from build123d import *

# Parameters (mm, degrees)
SKETCH10_R              = 7.4
SKETCH10_R_2            = 4.5
BOSS_EXTRUDE3_DEPTH     = 1.2
SKETCH11_R              = 7.4
SKETCH11_R_2            = 5.2
BOSS_EXTRUDE4_DEPTH     = 20
BOSS_EXTRUDE5_DEPTH     = 7
SKETCH12_R              = 0.75
CUT_EXTRUDE1_DEPTH      = 10
CUT_EXTRUDE1_DEPTH_BACK = 11
SKETCH14_W              = 4.2
SKETCH14_H              = 1
CUT_EXTRUDE2_DEPTH      = 6
CUT_EXTRUDE3_REACH      = 29.148
CUT_EXTRUDE3_END_RADIUS = 7.4
CUT_EXTRUDE6_DEPTH      = 1
SKETCH16_R              = 0.8
CUT_EXTRUDE4_DEPTH      = 10
CUT_EXTRUDE4_DEPTH_BACK = 10
SKETCH19_R              = 7.4
SKETCH19_R_2            = 7
CUT_EXTRUDE7_DEPTH      = 15.2
FILLET1_R               = 1


with BuildPart() as part:
    # Sketch10 → Boss-Extrude3 (new body)
    with BuildSketch(Plane.XY):
        Circle(SKETCH10_R)
        Circle(SKETCH10_R_2, mode=Mode.SUBTRACT)
    extrude(amount=BOSS_EXTRUDE3_DEPTH)

    # Sketch11 → Boss-Extrude4 (add)
    with BuildSketch(Plane(origin=(0, 0, 0), x_dir=(-1, 0, 0), z_dir=(0, 0, -1))):
        Circle(SKETCH11_R)
        Circle(SKETCH11_R_2, mode=Mode.SUBTRACT)
    extrude(amount=BOSS_EXTRUDE4_DEPTH)

    # Sketch13 → Boss-Extrude5 (add)
    with BuildSketch(Plane.XY.offset(1.2)):
        with BuildLine():
            ThreePointArc((-2.9, 6.808083431), (0, 7.4), (2.9, 6.808083431))
            Line((2.9, 6.808083431), (2.9, 8.4))
            Line((2.9, 8.4), (-2.9, 8.4))
            Line((-2.9, 8.4), (-2.9, 6.808083431))
        make_face()
        with BuildLine():
            ThreePointArc((2.9, -6.808083431), (0, -7.4), (-2.9, -6.808083431))
            Line((-2.9, -6.808083431), (-2.9, -8.4))
            Line((-2.9, -8.4), (2.9, -8.4))
            Line((2.9, -8.4), (2.9, -6.808083431))
        make_face()
    extrude(amount=-BOSS_EXTRUDE5_DEPTH)

    # Sketch12 → Cut-Extrude1 (cut, two sides)
    with BuildSketch(Plane(origin=(0, 0, 0), x_dir=(1, 0, 0), z_dir=(0, 1, 0))) as cut_extrude1_sk:
        with Locations(Location((0, 1.8, 0), (0, 0, 90))):
            Circle(SKETCH12_R)
    extrude(amount=CUT_EXTRUDE1_DEPTH, mode=Mode.SUBTRACT)
    extrude(cut_extrude1_sk.sketch, amount=-CUT_EXTRUDE1_DEPTH_BACK, mode=Mode.SUBTRACT)

    # Sketch14 → Cut-Extrude2 (cut)
    with BuildSketch(Plane.XY.offset(1.2)):
        with Locations((0, 7.9)):
            Rectangle(SKETCH14_W, SKETCH14_H)
        with Locations((0, -7.9)):
            Rectangle(SKETCH14_W, SKETCH14_H)
    extrude(amount=-CUT_EXTRUDE2_DEPTH, mode=Mode.SUBTRACT)

    # Cut-Extrude3: up to this cylinder (the profile starts outside it)
    cut_extrude3_end = Plane(origin=(0, 0, -5.3), z_dir=(0, 0, -1)) * Cylinder(CUT_EXTRUDE3_END_RADIUS, 74.096, mode=Mode.PRIVATE)
    # Sketch15 → Cut-Extrude3 (cut, up to the surface)
    with BuildSketch(Plane(origin=(0, 8.4, 0), x_dir=(1, 0, 0), z_dir=(0, 1, 0)), mode=Mode.PRIVATE) as cut_extrude3_sk1:
        Polygon((-2.9, 5.8), (-2.9, 4.8), (-2.1, 4.8), (2.1, 4.8), (2.9, 4.8), (2.9, 5.8), align=None)
    cut_extrude3_tool1 = extrude(cut_extrude3_sk1.sketch, amount=-CUT_EXTRUDE3_REACH, mode=Mode.PRIVATE) - cut_extrude3_end
    add(cut_extrude3_tool1.solids().sort_by_distance((0, 8.4, -5.3))[0], mode=Mode.SUBTRACT)

    # Sketch18 → Cut-Extrude6 (cut)
    with BuildSketch(Plane(origin=(0, 0, -5.8), x_dir=(-1, 0, 0), z_dir=(0, 0, -1))):
        with BuildLine():
            Line((-2.9, -6.808083431), (-2.9, -8.4))
            Line((-2.9, -8.4), (2.9, -8.4))
            Line((2.9, -8.4), (2.9, -6.808083431))
            ThreePointArc((2.9, -6.808083431), (0, -7.4), (-2.9, -6.808083431))
        make_face()
    extrude(amount=-CUT_EXTRUDE6_DEPTH, mode=Mode.SUBTRACT)

    # Sketch16 → Cut-Extrude4 (cut, two sides)
    with BuildSketch(Plane(origin=(0, 0, 0), x_dir=(0, 0, -1), z_dir=(1, 0, 0))) as cut_extrude4_sk:
        with Locations(Location((15, 0, 0), (0, 0, 180))):
            Circle(SKETCH16_R)
    extrude(amount=CUT_EXTRUDE4_DEPTH, mode=Mode.SUBTRACT)
    extrude(cut_extrude4_sk.sketch, amount=-CUT_EXTRUDE4_DEPTH_BACK, mode=Mode.SUBTRACT)

    # Sketch19 → Cut-Extrude7 (cut)
    with BuildSketch(Plane(origin=(0, 0, -20), x_dir=(-1, 0, 0), z_dir=(0, 0, -1))):
        Circle(SKETCH19_R)
        Circle(SKETCH19_R_2, mode=Mode.SUBTRACT)
    extrude(amount=-CUT_EXTRUDE7_DEPTH, mode=Mode.SUBTRACT)

    # Fillet1
    fillet1_edges = [part.edges().sort_by_distance(p)[0] for p in [
        (7, 0, -20),
    ]]
    fillet(fillet1_edges, radius=FILLET1_R)


solid = part.part
Check sheet for the modelled part. Datum: model origin and axes. Units: mm. A direction names the side the tool comes from. Round coordinates to 2 decimals unless told otherwise and drop trailing zeros. Loops run counter-clockwise (first coordinate to the right, second up) from the corner with the lowest first, then second, coordinate; pieces in that order, holes last.
1. Sectioned sample at C-C on y = 0. Record the boundary of the cut face in (x, z), and give its area (3 significant figures).
2. Mould release check, pull along X, two halves, no side actions. Record for faces 6 (the cylindrical face through (-0.59, 4.46, 0.59)), 7 (the flat face through (-2.9, 8, -2)), 8 (the flat face through (2.9, 8, -2)), 9 (the flat face through (2, 5, -20)): released by +X, released by -X, zero draft, split by the parting line, or undercut.
3. Sectioned sample at B-B on z = -1.8. Record the boundary of the cut face in (x, y).
4. Set-up check for faces 1 (the flat face through (-2.1, -8, -2)), 2 (the flat face through (2.9, -8, -2)), 3 (the flat face through (-2.1, 8, -2)), 4 (the flat face through (-2.9, -8, -2)), 5 (the cylindrical face through (-4.96, 1.56, -9.86)): record each of +Z, -Z, +X, -X, +Y, -Y from which the full face is reachable in a straight line by a thin tool's end or side.
5. Gauge pin test, flat ends, axial feed: pin 1 Ø3.5 at (x, z) = (1, -1.5) entering from -Y; pin 2 Ø1.3 at (y, z) = (7.5, -3) entering from -X; pin 3 Ø0.8 at (y, z) = (7.5, -0.5) entering from +X; pin 4 Ø1.7 at (x, z) = (0, -1.8) entering from +Y. Record the tip position at first contact, or that the pin passes through.
6. Sectioned sample at A-A on x = 0. Record the boundary of the cut face in (y, z), and give its area (3 significant figures).
7. Sectioned sample at D-D on z = -4.5. Record the boundary of the cut face in (x, y).
8. Scan lines: probe 1 along Y at (x, z) = (0, 0.35); probe 2 along Y at (x, z) = (0, -4.5); probe 3 along Z at (x, y) = (4, 3). Record each from-to range of solid material in increasing order.
Recorded:
1. outline: (-7.4, -4.8) - (-7, -4.8) - (-7, -14.2) - (-5.2, -14.2) - (-5.2, 0) - (-4.5, 0) - (-4.5, 1.2) - (-7.4, 1.2) - close; (-7, -19) arc R1 ccw to (-6, -20) - (-5.2, -20) - (-5.2, -15.8) - (-7, -15.8) - close; (4.5, 0) - (5.2, 0) - (5.2, -14.2) - (7, -14.2) - (7, -4.8) - (7.4, -4.8) - (7.4, 1.2) - (4.5, 1.2) - close; (5.2, -20) - (6, -20) arc R1 ccw to (7, -19) - (7, -15.8) - (5.2, -15.8) - close
1. area: 76.6 mm2
2. face 6: undercut
2. face 7: released by -X
2. face 8: released by +X
2. face 9: zero draft
3. outline: (-2.9, -8.4) - (-2.1, -8.4) - (-2.1, -7.4) - (-0.75, -7.4) - (-0.75, -5.15) arc R5.2 cw to (-0.75, 5.15) - (-0.75, 7.4) - (-2.1, 7.4) - (-2.1, 8.4) - (-2.9, 8.4) - (-2.9, 6.81) arc R7.4 ccw to (-2.9, -6.81) - close; (0.75, -7.4) - (2.1, -7.4) - (2.1, -8.4) - (2.9, -8.4) - (2.9, -6.81) arc R7.4 ccw to (2.9, 6.81) - (2.9, 8.4) - (2.1, 8.4) - (2.1, 7.4) - (0.75, 7.4) - (0.75, 5.15) arc R5.2 cw to (0.75, -5.15) - close
4. face 1: +Z, -Z, -Y
4. face 2: +Z, -Z, +X, -Y
4. face 3: +Z, -Z, +Y
4. face 4: +Z, -Z, -X, -Y
4. face 5: -Z
5. pin 1: stops at y = -8.4
5. pin 2: stops at x = -2.9
5. pin 3: stops at x = 2.9
5. pin 4: stops at y = 7.4
6. outline: (-7.4, -4.8) - (-7, -4.8) - (-7, -19) arc R1 ccw to (-6, -20) - (-5.2, -20) - (-5.2, -2.55) - (-7.4, -2.55) - close; (-7.4, -1.05) - (-5.2, -1.05) - (-5.2, 0) - (-4.5, 0) - (-4.5, 1.2) - (-7.4, 1.2) - close; (4.5, 0) - (5.2, 0) - (5.2, -1.05) - (7.4, -1.05) - (7.4, 1.2) - (4.5, 1.2) - close; (5.2, -20) - (6, -20) arc R1 ccw to (7, -19) - (7, -4.8) - (7.4, -4.8) - (7.4, -2.55) - (5.2, -2.55) - close
6. area: 75.8 mm2
7. outline: (-2.9, -8.4) - (-2.1, -8.4) - (-2.1, -7.4) - (2.1, -7.4) - (2.1, -8.4) - (2.9, -8.4) - (2.9, -6.81) arc R7.4 ccw to (2.9, 6.81) - (2.9, 8.4) - (2.1, 8.4) - (2.1, 7.4) - (-2.1, 7.4) - (-2.1, 8.4) - (-2.9, 8.4) - (-2.9, 6.81) arc R7.4 ccw to (-2.9, -6.81) - close; hole circle Ø10.4 at (0, 0)
8. probe 1: y = -7.4 to -4.5, 4.5 to 7.4
8. probe 2: y = -7.4 to -5.2, 5.2 to 7.4
8. probe 3: z = 0 to 1.2
